Source: CAD feature listing. Evaluate the final solid. Frame: model axes, mm. A direction names the side the tool comes from. Coordinates: 2 decimals unless noted, no trailing zeros. Loops run counter-clockwise (first coordinate to the right, second up) from the corner with the lowest first, then second, coordinate; pieces in that order, holes last. Notation, with made-up numbers: (-38, 29) - (-17, 29) arc R6 ccw to (-17, 35) - close; hole circle Ø11 at (34.5, 79). An arc over 180 degrees is marked (long way). Use one line per item in the form item = value. Start each with the question number.
Autodesk Inventor part; units mm, degrees
ref_plane "YZ Plane" through (0, 0, 0) normal (1, 0, 0) x (0, 1, 0)
ref_plane "XZ Plane" through (0, 0, 0) normal (0, 1, 0) x (-1, 0, 0)
ref_plane "XY Plane" through (0, 0, 0) normal (0, 0, 1) x (1, 0, 0)
sketch "Sketch1" plane through (0, 0, 0) normal (0, 1, 0) x (-1, 0, 0)
  line L0 (0, 0) -> (0, -2.8284)
  line L1 (0, -2.8284) -> (29, 26.1716)
  line L2 (29, 26.1716) -> (29, 29)
  line L3 (29, 29) -> (0, 0)
  line L4 (29, 26.1716) -> (35, 32.1716)
  line L5 (35, 32.1716) -> (35, 35)
  line L6 (35, 35) -> (29, 29)
  dimension "d2" = 29
  dimension "d3" = 45
  dimension "d6" = 2
  dimension "d23" = 6
  dimension "d24" = 45
  dimension "d25" = 45
extrude "Extrusion1" add sketch "Sketch1" along normal mid plane 100 contours L3 L2 L1 L0
sketch "Sketch2" plane through (0, 0, 0) normal (0, 0, 1) x (1, 0, 0)
  line L0 (-17, 36) -> (-6, 36)
  line L1 (-6, 36) -> (-6, 19)
  line L2 (-6, 19) -> (-17, 19)
  line L3 (-17, 19) -> (-17, 36)
  line L4 (0, 50) -> (-29, 50)
  line L5 (0, -50) -> (0, 50)
  point P0 (0, 0)
  dimension "d7" = 14
  dimension "d8" = 17
  dimension "d9" = 11
  dimension "d11" = 6
extrude "Extrusion2" cut sketch "Sketch2" along normal up to next
mirror "Mirror1" about plane through (0, 0, 0) normal (0, 1, 0) of "Extrusion2"
sketch "Sketch3" plane through (0, -50, 0) normal (0.7071, 0, 0.7071) x (0.7071, 0, -0.7071)
  circle A0 centre (-30.5122, 5) radius 1.25
  circle A1 centre (-15.5122, 5) radius 1.25
  line L0 (-39.0122, 0) -> (-39.0122, 100)
  line L1 (-41.0122, 0) -> (-41.0122, 100)
  line L2 (0, 0) -> (-41.0122, 0)
  point P0 (0, 50)
  dimension "d15" = 5
  dimension "d16" = 2.5
  dimension "d17" = 15
  dimension "d18" = 2.5
  dimension "d19" = 5
  dimension "d20" = 10.5
extrude "Extrusion3" cut sketch "Sketch3" against normal up to next
mirror "Mirror2" about plane through (0, 0, 0) normal (0, 1, 0) of "Extrusion3"
extrude "Extrusion4" add sketch "Sketch1" along normal mid plane 100 contours L6 L5 L4 L2
properties part number "Front_Dluzszy_2"
(1) Mould query, pull axis Z, two halves, no side actions, for faces 4 (the face through (-11.78, -43.76, 10.39)), 5 (the face through (-17.26, -0.7, 14.43)), 6 (the face through (-12, 36, 10)). Classes: +Z half, -Z half, draft (parallel to the pull), parting line (faces both ways), or undercut.
(2) Cut plane B-B, the plane z = 28. Output: boundary loops of the cut face in (x, y).
(3) Material intervals for line 1 (X direction, y = -5, z = 24.5); line 2 (Z direction, x = -25, y = -21.5); line 3 (Z direction, x = -13, y = -4), sorted ascending.
(4) Access query for faces 1 (the face through (-18, -1, 18)), 2 (the face through (-17, -28, 16)), 3 (the face through (-6, -27, 5)). Directions: +Z, -Z, +X, -X, +Y, -Y. A direction counts if a zero-diameter tool reaches every point of the face in a straight line with its end or side. Return the directions, or none.
(5) Contact query for flat-ended pins moving along their axis: pin 1 (4 mm diameter, centred on y = -9.5, z = 26, fed in from +X); pin 2 (12 mm diameter, centred on y = -29, z = 24.5, fed in from -X); pin 3 (2 mm diameter, centred on x = -21.5, y = 2.5, fed in from -Z); pin 4 (2 mm diameter, centred on x = -20, z = 14, fed in from +Y). Output: stop coordinate, or through.
(6) Cut plane A-A, the plane y = -21. Output: boundary loops of the cut face in (x, z).
(7) Cut plane C-C, the plane x = -4. Output: boundary loops of the cut face in (y, z), plus the area to 3 significant figures.
Recorded:
q1.face_4 = undercut
q1.face_5 = -Z half
q1.face_6 = draft
q2.outline = (-30.83, -50) - (-28, -50) - (-28, 50) - (-30.83, 50) - close
q3.line_1 = -27.33 to -24.5
q3.line_2 = 22.17 to 25
q3.line_3 = 10.17 to 13
q4.face_1 = +Z, +X, +Y, -Y
q4.face_2 = +Z, -Z, +X
q4.face_3 = +Z, -Z, -X
q5.pin_1 = -24
q5.pin_2 = -33.33
q5.pin_3 = 17.67
q5.pin_4 = through
q6.outline = (-35, 32.17) - (-17, 14.17) - (-17, 17) - (-35, 35) - close; (-6, 3.17) - (0, -2.83) - (0, 0) - (-6, 6) - close
q7.outline = (-50, 1.17) - (50, 1.17) - (50, 4) - (-50, 4) - close
q7.area = 283 mm²
